For this review, take the finished solid that the model builds, in its own axes (mm). A direction names the side the tool comes from. Round coordinates to 2 decimals unless told otherwise and drop trailing zeros. Order: outer loops, then holes, each group sorted by start corner. A loop starts at its lowest first (then second) coordinate and runs counter-clockwise, first axis right, second up. Notation, with made-up numbers: (45, 83) -> (49, 83) arc R16 ccw to (49, 112) -> close; hole circle Ø11 at (-34.75, -4). An arc over 180 degrees is marked (long way). Put each result on its own line as item: value. Start each with the question number.
```python
from build123d import *

# Parameters (mm, degrees)
SKETCH1_W           = 61.9125
SKETCH1_H           = 22.225
BOSS_EXTRUDE1_DEPTH = 34.925
SKETCH2_W           = 22.225
SKETCH2_H           = 28.575
BOSS_EXTRUDE2_DEPTH = 28.575
SKETCH3_W           = 28.575
SKETCH3_H           = 22.225
BOSS_EXTRUDE3_DEPTH = 28.575
SKETCH4_R           = 9.525
BOSS_EXTRUDE4_DEPTH = 19.05
SKETCH5_R           = 6.35
BOSS_EXTRUDE5_DEPTH = 6.35
FILLET1_R           = 3.81


with BuildPart() as part:
    # Sketch1 → Boss-Extrude1 (new body)
    with BuildSketch(Plane(origin=(0, 0, 0), x_dir=(1, 0, 0), z_dir=(0, 1, 0))):
        with Locations((30.95625, 11.1125)):
            Rectangle(SKETCH1_W, SKETCH1_H)
    extrude(amount=BOSS_EXTRUDE1_DEPTH)

    # Sketch2 → Boss-Extrude2 (add)
    with BuildSketch(Plane.ZY):
        with Locations((-11.1125, 20.6375)):
            Rectangle(SKETCH2_W, SKETCH2_H)
    extrude(amount=BOSS_EXTRUDE2_DEPTH)

    # Sketch3 → Boss-Extrude3 (add)
    with BuildSketch(Plane(origin=(0, 34.925, 0), x_dir=(1, 0, 0), z_dir=(0, 1, 0))):
        with Locations((-14.2875, 11.1125)):
            Rectangle(SKETCH3_W, SKETCH3_H)
    extrude(amount=BOSS_EXTRUDE3_DEPTH)

    # Sketch4 → Boss-Extrude4 (add)
    with BuildSketch(Plane(origin=(0, 0, 0), x_dir=(0, 0, -1), z_dir=(1, 0, 0))):
        with Locations(Location((11.1125, 53.975, 0), (0, 0, 90))):
            Circle(SKETCH4_R)
    extrude(amount=BOSS_EXTRUDE4_DEPTH)

    # Sketch5 → Boss-Extrude5 (add)
    with BuildSketch(Plane.ZY.offset(28.575)):
        with Locations((-11.1125, 15.875)):
            Circle(SKETCH5_R)
    extrude(amount=BOSS_EXTRUDE5_DEPTH)

    # Fillet1
    fillet1_edges = [part.edges().sort_by_distance(p)[0] for p in [
        (-14.2875, 6.35, -22.225),
        (-14.2875, 6.35, 0),
    ]]
    fillet(fillet1_edges, radius=FILLET1_R)


solid = part.part
```
Item 1: Consider section C-C, the plane y = 51.5. Write out the cut boundary in (x, z) (3 decimals).
Item 2: Mouldability with a two-part tool opening along Y and no side actions: class faces 1 (the face through (-14.49, 7.5, -21.14)), 2 (the face through (9.39, 44.46, -10.69)), 3 (the face through (16, 24, -22.225)), 4 (the face through (0, 43, -11)) as +Y half, -Y half, draft (parallel to the pull), parting line (faces both ways), or undercut.
Item 3: Consider section D-D, the plane x = 28.5. Write out the cut boundary in (y, z) (3 decimals).
Item 4: Tool access review of faces 5 (the face through (-14, 6.35, -11)), 6 (the face through (19.05, 54, -11)), 7 (the face through (-14.488, 7.496, -1.086)), 8 (the face through (31, 34.925, -11)): name each direction out of +Z, -Z, +X, -X, +Y, -Y from which nothing blocks a thin tool from reaching the whole face with its end or side.
Item 5: For L1, parallel to Y at x = -18, z = -4; L2, parallel to X at y = 31.5, z = -3.25 (1 decimal); L3, parallel to Y at x = 39, z = -4.25 (3 decimals), list the stretches that pass through material, from the lowest coordinate up.
Item 6: Insertion check: pin 1 Ø11 at (y, z) = (48, -12) entering from -X (3 decimals); pin 2 Ø7.5 at (x, z) = (-14.5, -14.5) entering from -Y; pin 3 Ø11 at (x, z) = (41, -14) entering from +Y (3 decimals). Each pin has a flat end and moves straight along its axis. Give the tip position at first contact, or say it passes through.
Evaluation:
1. outline: (-28.575, -22.225) -> (0, -22.225) -> (0, -20.31) -> (19.05, -20.31) -> (19.05, -1.915) -> (0, -1.915) -> (0, 0) -> (-28.575, 0) -> close
2. face 1: -Y half
2. face 2: undercut
2. face 3: draft
2. face 4: undercut
3. outline: (0, -22.225) -> (34.925, -22.225) -> (34.925, 0) -> (0, 0) -> close
4. face 5: +Z, -Z, -X, -Y
4. face 6: +Z, -Z, +X, +Y
4. face 7: +Z, -X, -Y
4. face 8: +Z, -Z, +X
5. L1: y = 6.35 to 63.5
5. L2: x = -28.6 to 61.9
5. L3: y = 0 to 34.925
6. pin 1: stops at x = -28.575
6. pin 2: stops at y = 6.35
6. pin 3: stops at y = 34.925
